Part print with two shaded views. Sizes in mm from the minimum x, y, z corner. Coordinates: 2 decimals unless noted, no trailing zeros. Loops run counter-clockwise (first coordinate to the right, second up) from the corner with the lowest first, then second, coordinate; pieces in that order, holes last.
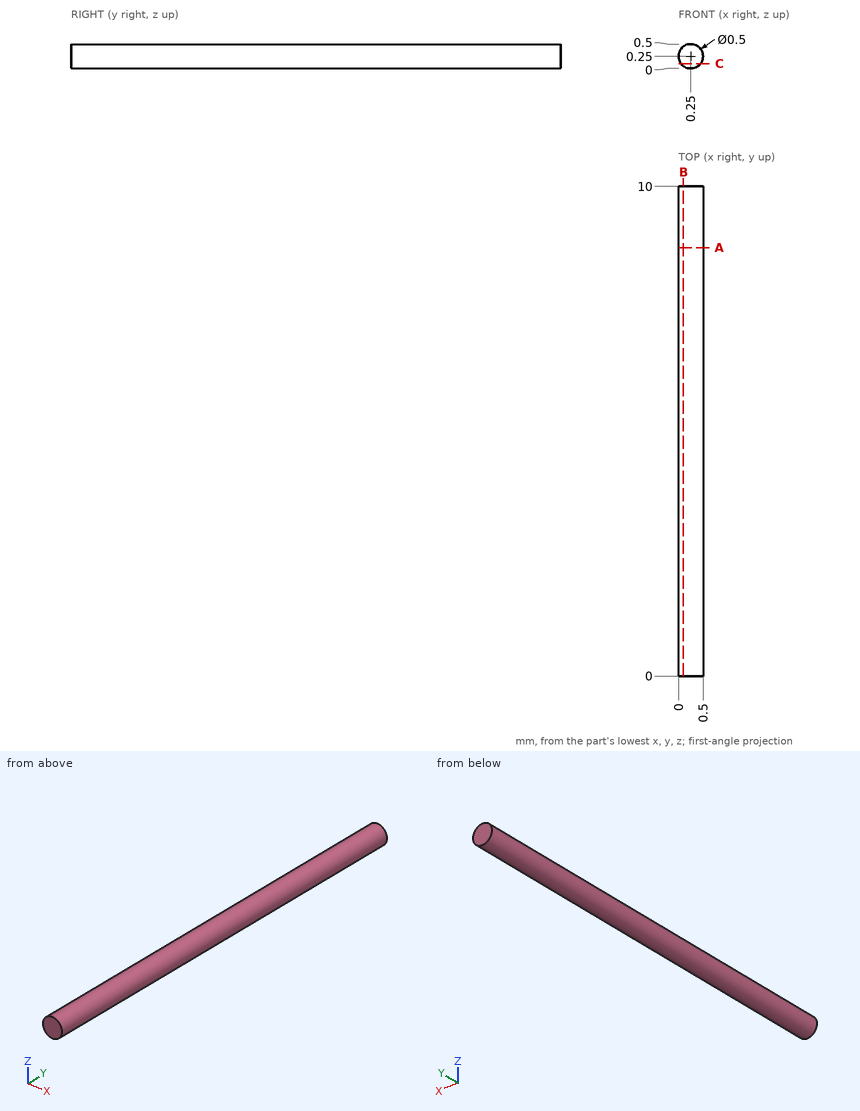
Q1. Slice it at A-A (y = 8.75). List the corners of the cut face in (x, z).
Answers:
outline: circle Ø0.5 at (0.25, 0.25)
Q2. Slice it at B-B (x = 0.1). List the corners of the cut face in (y, z), and give its area (3 significant figures).
Answers:
outline: (0, 0.05) - (10, 0.05) - (10, 0.45) - (0, 0.45) - close
area: 4.00 mm2
Q3. Drill centre lines: line 1 (X direction, y = 2, z = 0.4); line 2 (Z direction, x = 0.35, y = 7.5). Where is each one in solid material? Low to high.
Answers:
line 1: x = 0.05 to 0.45
line 2: z = 0.02 to 0.48
Q4. Slice it at C-C (z = 0.1). List the corners of the cut face in (x, y), and give its area (3 significant figures).
Answers:
outline: (0.05, 0) - (0.45, 0) - (0.45, 10) - (0.05, 10) - close
area: 4.00 mm2
